Geometry: final body of the model. Coordinates: model frame, mm. Round coordinates to 2 decimals unless told otherwise and drop trailing zeros. Loops run counter-clockwise (first coordinate to the right, second up) from the corner with the lowest first, then second, coordinate; pieces in that order, holes last. Notation, with made-up numbers: (-17.75, 26.25) - (-11.75, 26.25) arc R21 cw to (-11.75, 57.25) - close; hole circle Ø6 at (1.5, -13). An arc over 180 degrees is marked (long way). Return JSON: item names as keys, results as strings. Group by question number.
1. Section B-B on y = 0. Return loops of the section in (x, z).
2. Section A-A on z = 0. Return loops of the section in (x, y).
3. Material intervals for probe 1 along Y at (x, z) = (7, 0); probe 2 along X at (y, z) = (0, 718), sorted ascending.
4. Section C-C on x = 0. Return loops of the section in (y, z).
5. Section D-D on z = 635. Return loops of the section in (x, y), and give its area (3 significant figures).
6. First-contact query: pin 1 Ø12 at (x, y) = (-4.5, 8.5) entering from +Z; pin 2 Ø10 at (x, z) = (-10, 196.5) entering from +Y; pin 3 Ø10 at (x, y) = (20, 14.5) entering from -Z. Flat tips, straight axial feed; report the tip coordinate or a pass-through.
from build123d import *

# Parameters (mm, degrees)
SKETCH_1_R          = 21
EXTRUDE_1_DEPTH     = 900
SKETCH_2_R          = 18
CUT_EXTRUDE_1_DEPTH = 901
SKETCH_4_R          = 30
EXTRUDE_2_DEPTH     = 30
SKETCH_5_R          = 25
CUT_EXTRUDE_2_DEPTH = 61.0000001


with BuildPart() as part:
    # Эскиз1 → Бобышка-Вытянуть1 (new body)
    with BuildSketch(Plane.XY):
        Circle(SKETCH_1_R)
    extrude(amount=EXTRUDE_1_DEPTH)

    # Эскиз2 → Вырез-Вытянуть1 (cut, through all)
    with BuildSketch(Plane(origin=(0, 0, 0), x_dir=(-1, 0, 0), z_dir=(0, 0, -1))):
        Circle(SKETCH_2_R)
    extrude(amount=-CUT_EXTRUDE_1_DEPTH, mode=Mode.SUBTRACT)

    # Эскиз4 → Бобышка-Вытянуть2 (add, symmetric)
    with BuildSketch(Plane(origin=(0, 0, 0), x_dir=(0, 0, -1), z_dir=(1, 0, 0))):
        Circle(SKETCH_4_R)
    extrude(amount=EXTRUDE_2_DEPTH, both=True)

    # Эскиз5 → Вырез-Вытянуть2 (cut, through all)
    with BuildSketch(Plane(origin=(30, 0, 0), x_dir=(0, 0, -1), z_dir=(1, 0, 0))):
        Circle(SKETCH_5_R)
    extrude(amount=-CUT_EXTRUDE_2_DEPTH, mode=Mode.SUBTRACT)


solid = part.part
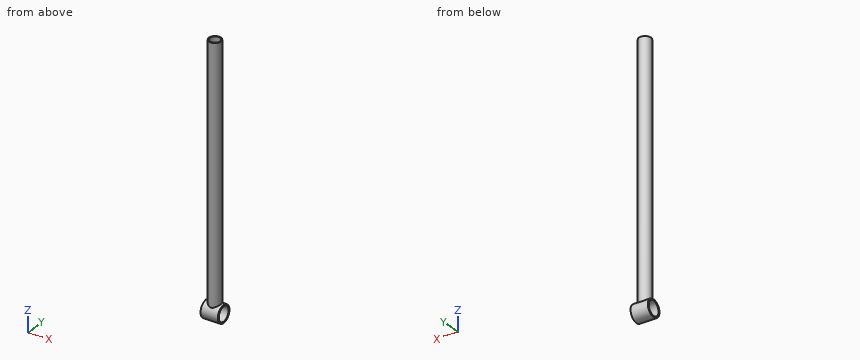
Taken from the geometry:
{
 "1": {"outline": "(-30, -30) - (30, -30) - (30, -25) - (-30, -25) - close; (-30, 25) - (30, 25) - (30, 30) - (21, 30) - (21, 900) - (18, 900) - (18, 30) - (-18, 30) - (-18, 900) - (-21, 900) - (-21, 30) - (-30, 30) - close"},
 "2": {"outline": "(-30, -30) - (30, -30) - (30, -25) - (-30, -25) - close; (-30, 25) - (30, 25) - (30, 30) - (-30, 30) - close"},
 "3": {"probe 1": "-30 to -25, 25 to 30", "probe 2": "-21 to -18, 18 to 21"},
 "4": {"outline": "(-21, 21.42) arc R30 ccw (long way) to (21, 21.42) - (21, 900) - (18, 900) - (18, 24) arc R30 ccw to (-18, 24) - (-18, 900) - (-21, 900) - close; hole circle Ø50 at (0, 0)"},
 "5": {"outline": "circle Ø42 at (0, 0); hole circle Ø36 at (0, 0)", "area": "368 mm2"},
 "6": {"pin 1": "z = 29.9", "pin 2": "y = 20.4", "pin 3": "z = -28.46"}
}
